Design review of the part built by this model. Coordinates are the model's own, in mm. Face numbers are marked on the shaded views. Round coordinates to 2 decimals unless told otherwise and drop trailing zeros. Write each loop counter-clockwise with the first axis right and the second up, starting at its lowest first coordinate (ties: lowest second). Pieces come first, ordered by that corner, then holes. Notation, with made-up numbers: (77.5, 73.25) -> (105.5, 73.25) arc R24 cw to (105.5, 94.25) -> close; hole circle Ø5 at (-21.5, 63.5). An arc over 180 degrees is marked (long way). One line per question, with ' | ' between items. Start each with the question number.
1) Mouldability with a two-part tool opening along X and no side actions: class the marked faces 1 and 2 as +X half, -X half, draft (parallel to the pull), parting line (faces both ways), or undercut.
2) Insertion check: pin 1 Ø2 at (x, z) = (-38, 36.5) entering from +Y. The pin has a flat end and moves straight along its axis. Give the tip position at first contact, or say it passes through.
3) For probe 1 along X at (y, z) = (3.75, 64.5); probe 2 along X at (y, z) = (1.75, 52.5); probe 3 along Y at (x, z) = (-16, 76), list the stretches that pass through material, from the lowest coordinate up.
4) Consider section B-B (z = 19.5). Give the boundary of the cut face in (x, y), then the cut area to 3 significant figures.
5) Consider section A-A (y = 6.5). Give the boundary of the cut face in (x, z).
6) Consider section C-C (x = -14.5). Give the boundary of the cut face in (y, z).
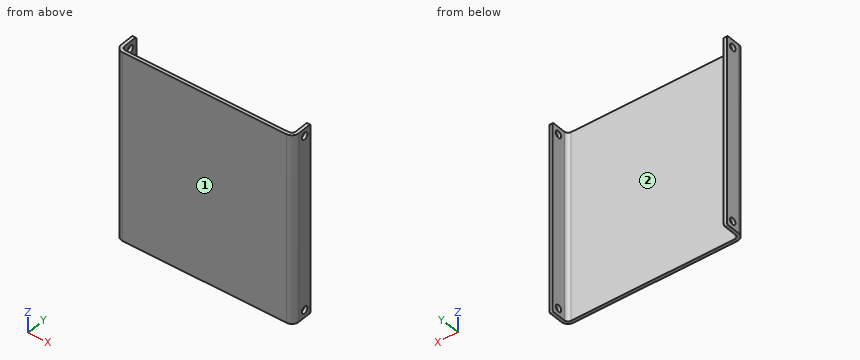
```python
from build123d import *

# Parameters (mm, degrees)
F1_DEPTH = 101.6
F2_R     = 3.69316
F3_R     = 1.98374
F4_R     = 1.8288
F5_DEPTH = 95.37192
F6_R     = 0.762


with BuildPart() as f1:
    # F0 (on Top) → F1 (new body)
    with BuildSketch(Plane.XY):
        Polygon((0, 9.92124), (0, 0), (-91.95308, 0), (-91.95308, 9.92124), (-93.6625, 9.92124), (-93.6625, -1.70942), (1.70942, -1.70942), (1.70942, 9.92124), align=None)
    extrude(amount=F1_DEPTH)

    # F2
    f2_edges = [f1.edges().sort_by_distance(p)[0] for p in [
        (1.70942, -1.70942, 50.8),
        (-93.6625, -1.70942, 50.8),
    ]]
    fillet(f2_edges, radius=F2_R)

    # F3
    f3_edges = [f1.edges().sort_by_distance(p)[0] for p in [
        (0, 0, 50.8),
        (-91.95308, 0, 50.8),
    ]]
    fillet(f3_edges, radius=F3_R)

    # F4 (on face) → F5 (cut, through all)
    with BuildSketch(Plane.YZ.offset(1.70942)):
        with Locations((5.95249, 97.63125)):
            Circle(F4_R)
        with Locations((5.95249, 3.96875)):
            Circle(F4_R)
    extrude(amount=-F5_DEPTH, mode=Mode.SUBTRACT)

    # F6
    f6_edges = [f1.edges().sort_by_distance(p)[0] for p in [
        (-92.80779, 9.92124, 101.6),
        (-92.80779, 9.92124, 0),
        (0.85471, 9.92124, 0),
        (0.85471, 9.92124, 101.6),
    ]]
    fillet(f6_edges, radius=F6_R)


solid = f1.part
```
From the geometry:
1) face 1: draft | face 2: undercut
2) pin 1: stops at y = 0
3) probe 1: x = -93.66 to -91.95, 0 to 1.71 | probe 2: x = -93.66 to -91.94, -0.01 to 1.7 | probe 3: y = -1.71 to 0
4) outline: (-93.66, 1.98) arc R3.69 ccw to (-89.97, -1.71) -> (-1.98, -1.71) arc R3.69 ccw to (1.71, 1.98) -> (1.71, 9.92) -> (0, 9.92) -> (0, 1.98) arc R1.98 cw to (-1.98, 0) -> (-89.97, 0) arc R1.98 cw to (-91.95, 1.98) -> (-91.95, 9.92) -> (-93.66, 9.92) -> close | area: 193 mm2
5) outline: (-93.66, 0) -> (-91.95, 0) -> (-91.95, 2.22) -> (-93.66, 2.22) -> close; (-93.66, 5.71) -> (-91.95, 5.71) -> (-91.95, 95.89) -> (-93.66, 95.89) -> close; (-93.66, 99.38) -> (-91.95, 99.38) -> (-91.95, 101.6) -> (-93.66, 101.6) -> close; (0, 0) -> (1.71, 0) -> (1.71, 2.22) -> (0, 2.22) -> close; (0, 5.71) -> (1.71, 5.71) -> (1.71, 95.89) -> (0, 95.89) -> close; (0, 99.38) -> (1.71, 99.38) -> (1.71, 101.6) -> (0, 101.6) -> close
6) outline: (-1.71, 0) -> (0, 0) -> (0, 101.6) -> (-1.71, 101.6) -> close
